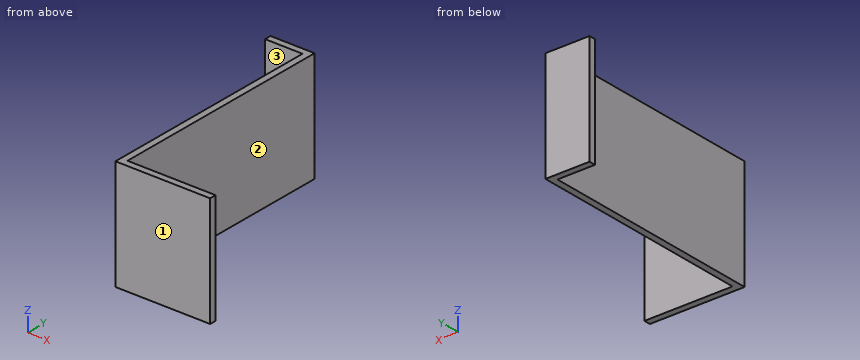
```python
from build123d import *

# Parameters (mm, degrees)
SKETCH1_W      = 43
SKETCH1_H      = 50
EXTRUDE1_DEPTH = 3
SKETCH2_W      = 3
SKETCH2_H      = 50
EXTRUDE2_DEPTH = 100
SKETCH3_W      = 20
SKETCH3_H      = 50
EXTRUDE3_DEPTH = 3


with BuildPart() as part:
    # Sketch1 → Extrude1 (new body)
    with BuildSketch(Plane(origin=(0, 0, 0), x_dir=(1, 0, 0), z_dir=(0, 1, 0))):
        with Locations((21.5, 25)):
            Rectangle(SKETCH1_W, SKETCH1_H)
    extrude(amount=EXTRUDE1_DEPTH)

    # Sketch2 → Extrude2 (add)
    with BuildSketch(Plane(origin=(0, 3, 0), x_dir=(1, 0, 0), z_dir=(0, 1, 0))):
        with Locations((1.5, 25)):
            Rectangle(SKETCH2_W, SKETCH2_H)
    extrude(amount=EXTRUDE2_DEPTH)

    # Sketch3 → Extrude3 (add)
    with BuildSketch(Plane(origin=(0, 103, 0), x_dir=(1, 0, 0), z_dir=(0, 1, 0))):
        with Locations((-7, 25)):
            Rectangle(SKETCH3_W, SKETCH3_H)
    extrude(amount=EXTRUDE3_DEPTH)


solid = part.part
```
CAD build for the part. Positions are in the model's coordinates, mm. Face numbers are marked on the shaded views. A direction names the side the tool comes from. Round coordinates to 2 decimals unless told otherwise and drop trailing zeros. Order: outer loops, then holes, each group sorted by start corner. A loop starts at its lowest first (then second) coordinate and runs counter-clockwise, first axis right, second up. Notation, with made-up numbers: (72.5, 55.5) - (98.5, 55.5) arc R8 cw to (98.5, 65.5) - close; hole circle Ø5 at (-4, -10.75). An arc over 180 degrees is marked (long way). Answer as CSV lines item,"result". Start each with the question number.
1. Saw through at B-B, the plane x = -2.5. Write the cut outline in (y, z).
2. Saw through at A-A, the plane z = -4. Write the cut outline in (x, y), and give its area (3 significant figures).
3. Tool access for the marked faces 1, 2 and 3: list every direction of +Z, -Z, +X, -X, +Y, -Y with a clear straight run to the whole face (end or side of a thin tool).
4. Pin check, flat tips, straight feed: pin 1 (2 mm diameter, centred on x = -4, z = -14.5, fed in from -Y); pin 2 (20 mm diameter, centred on x = 24.5, z = -32, fed in from +Y); pin 3 (10 mm diameter, centred on y = 37, z = -25.5, fed in from -X); pin 4 (5 mm diameter, centred on x = 0, z = -24.5, fed in from -Y). Stop position of each tip, or through.
5. Saw through at C-C, the plane y = 58. Write the cut outline in (x, z), and give its area (3 significant figures).
6. Drill centre lines: L1, parallel to Y at x = -13.5, z = -37; L2, parallel to Y at x = 26.5, z = -14. Where is each one in solid material? Low to high. Write a range as [from, to].
Model answer:
1,outline,"(103, -50) - (106, -50) - (106, 0) - (103, 0) - close"
2,outline,"(-17, 103) - (0, 103) - (0, 0) - (43, 0) - (43, 3) - (3, 3) - (3, 106) - (-17, 106) - close"
2,area,"489 mm²"
3,face 1,"+Z, -Z, +X, -X, -Y"
3,face 2,"+Z, -Z, +X, +Y"
3,face 3,"+Z, -Z, -X, -Y"
4,pin 1,"stops at y = 103"
4,pin 2,"stops at y = 3"
4,pin 3,"stops at x = 0"
4,pin 4,"stops at y = 0"
5,outline,"(0, -50) - (3, -50) - (3, 0) - (0, 0) - close"
5,area,"150 mm²"
6,L1,"y = [103, 106]"
6,L2,"y = [0, 3]"
